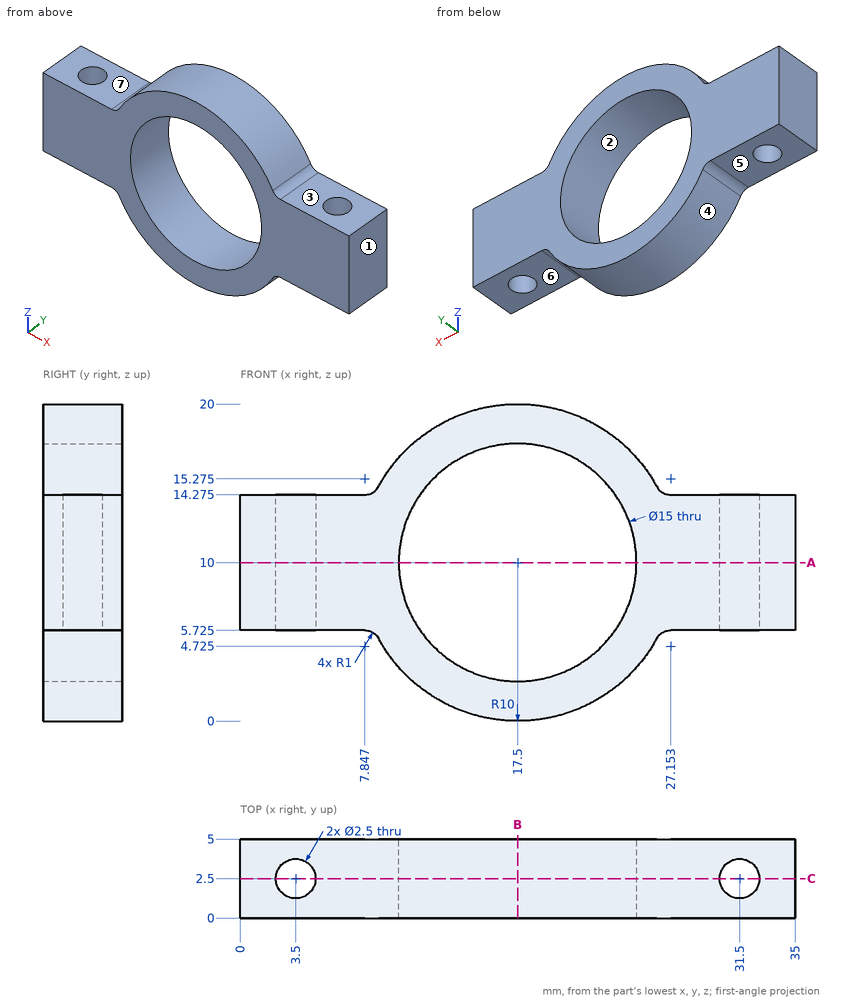
Job drawing, mm, ordinate dimensions from the low corner. One solid piece. A direction names the side the tool comes from. Give positions to 0.01 mm unless a question says otherwise; leave off trailing zeros. Write each loop counter-clockwise with the first axis right and the second up, starting at its lowest first coordinate (ties: lowest second). Pieces come first, ordered by that corner, then holes. Notation, with made-up numbers: (39.5, -10) - (63.5, -10) arc R25 ccw to (63.5, 26) - close; hole circle Ø9 at (51, -39). An arc over 180 degrees is marked (long way). Use one line per item in the form item = value. Start each with the question number.
1. Two-plate mould, pull along Z, no slides. Class the marked faces 1, 2, 3 and 4: released by +Z, released by -Z, zero draft, split by the parting line, or undercut.
2. Band-saw the part on C-C on y = 2.5. Count the separate pieces of the cut face and the enclosed holes in it.
3. Probe line 1 (Y direction, x = 31.5, z = 9.5); line 2 (Z direction, x = 28, y = 4) (1 decimal); line 3 (X direction, y = 2.6, z = 9.25). List the from-to ranges inside material, lowest first. Write a range as [from, to].
4. 3-axis set-ups, long thin cutter, end or side, ignore diameter. For the marked faces 5, 6 and 7: which of +Z, -Z, +X, -X, +Y, -Y reach the whole face in a straight line?
5. Drop flat-ended pins along their axis: pin 1 Ø1.5 at (x, y) = (30.5, 3) entering from +Z (3 decimals); pin 2 Ø12 at (x, z) = (17.5, 10) entering from +Y; pin 3 Ø1.5 at (x, y) = (32, 2) entering from -Z (3 decimals). Give the stop position or say it passes through.
6. Band-saw the part on A-A on z = 10. Write the cut outline in (x, y).
7. Band-saw the part on B-B on x = 17.5. Write the cut outline in (y, z), plus the area to 3 significant figures.
Conclusion:
q1.face_1 = zero draft
q1.face_2 = undercut
q1.face_3 = released by +Z
q1.face_4 = released by -Z
q2.separate_pieces = 3
q2.enclosed_holes = 1
q3.line_1 = [0, 1.25], [3.75, 5]
q3.line_2 = [5.7, 14.3]
q3.line_3 = [0, 2.25], [4.75, 10.04], [24.96, 30.25], [32.75, 35]
q4.face_5 = -Z, -X, +Y, -Y
q4.face_6 = -Z, +X, +Y, -Y
q4.face_7 = +Z, -X, +Y, -Y
q5.pin_1 = 14.275
q5.pin_2 = through
q5.pin_3 = 5.725
q6.outline = (0, 0) - (10, 0) - (10, 5) - (0, 5) - close; (25, 0) - (35, 0) - (35, 5) - (25, 5) - close; hole circle Ø2.5 at (3.5, 2.5); hole circle Ø2.5 at (31.5, 2.5)
q7.outline = (0, 0) - (5, 0) - (5, 2.5) - (0, 2.5) - close; (0, 17.5) - (5, 17.5) - (5, 20) - (0, 20) - close
q7.area = 25.0 mm²
